```python
from build123d import *

# Parameters (mm, degrees)
SKETCH1_W           = 23
SKETCH1_H           = 23
BOSS_EXTRUDE1_DEPTH = 4
SKETCH2_W           = 11
SKETCH2_H           = 11
CUT_EXTRUDE1_DEPTH  = 4
SKETCH3_W           = 9
SKETCH3_H           = 4
BOSS_EXTRUDE2_DEPTH = 30


with BuildPart() as part:
    # Sketch1 → Boss-Extrude1 (new body)
    with BuildSketch(Plane(origin=(0, 0, 0), x_dir=(1, 0, 0), z_dir=(0, 1, 0))):
        with Locations((-0.318811881, 0.227722772)):
            Rectangle(SKETCH1_W, SKETCH1_H)
    extrude(amount=BOSS_EXTRUDE1_DEPTH)

    # Sketch2 → Cut-Extrude1 (cut)
    with BuildSketch(Plane(origin=(0, 4, 0), x_dir=(1, 0, 0), z_dir=(0, 1, 0))):
        with Locations((-0.318811881, 0.227722772)):
            Rectangle(SKETCH2_W, SKETCH2_H)
    extrude(amount=-CUT_EXTRUDE1_DEPTH, mode=Mode.SUBTRACT)

    # Sketch3 → Boss-Extrude2 (add)
    with BuildSketch(Plane(origin=(11.181188119, 0, 0), x_dir=(0, 0, -1), z_dir=(1, 0, 0))):
        with Locations((0.227722772, 2)):
            Rectangle(SKETCH3_W, SKETCH3_H)
    extrude(amount=BOSS_EXTRUDE2_DEPTH)


solid = part.part
```
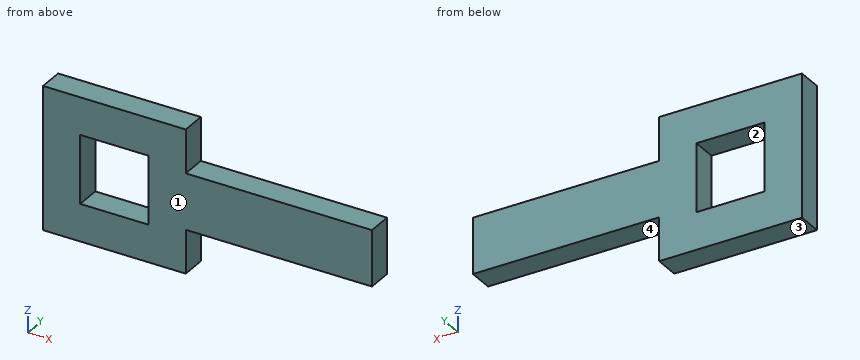
Work out the finished part from the listing and answer in its coordinate system (mm). Face numbers are marked on the shaded views. A direction names the side the tool comes from. Coordinates: 2 decimals unless noted, no trailing zeros. Write each loop counter-clockwise with the first axis right and the second up, starting at its lowest first coordinate (ties: lowest second). Pieces come first, ordered by that corner, then holes.
Q1. Determine the mould class of the marked faces 1 and 2 for opening direction X: released by +X, released by -X, zero draft, split by the parting line, or undercut.
Q2. A cutting plane is placed at D-D, the plane x = 36. Give the vertices of the cut face in (y, z).
Q3. A cutting plane is placed at C-C, the plane x = 1.5. Give the vertices of the cut face in (y, z).
Q4. This flat-tipped pin is pushed along its axis until it touches: pin 1 Ø1.2 at (x, y) = (30.5, 1) entering from -Z. Where does it stop, or does it pass through?
Q5. Which of the six approach directions +Z, -Z, +X, -X, +Y, -Y give full straight-line access (tool end or side, diameter ignored) to the marked faces 3 and 4?
Q6. A cutting plane is placed at A-A, the plane z = 2. Give the vertices of the cut face in (x, y).
Q7. A cutting plane is placed at B-B, the plane y = 0.7. Give the vertices of the cut face in (x, z).
Q8. Find the intervals of material crossed by line 1 (X direction, y = 1.95, z = -1.25); line 2 (Z direction, x = -2, y = 2.4); line 3 (X direction, y = 0.25, z = -5.25), in increasing order.
Findings below:
1. face 1: zero draft
1. face 2: undercut
2. outline: (0, -4.73) - (4, -4.73) - (4, 4.27) - (0, 4.27) - close
3. outline: (0, -11.73) - (4, -11.73) - (4, -5.73) - (0, -5.73) - close; (0, 5.27) - (4, 5.27) - (4, 11.27) - (0, 11.27) - close
4. pin 1: stops at z = -4.73
5. face 3: -Z, +X, -X, +Y, -Y
5. face 4: -Z, +X, +Y, -Y
6. outline: (-11.82, 0) - (-5.82, 0) - (-5.82, 4) - (-11.82, 4) - close; (5.18, 0) - (41.18, 0) - (41.18, 4) - (5.18, 4) - close
7. outline: (-11.82, -11.73) - (11.18, -11.73) - (11.18, -4.73) - (41.18, -4.73) - (41.18, 4.27) - (11.18, 4.27) - (11.18, 11.27) - (-11.82, 11.27) - close; hole (-5.82, -5.73) - (5.18, -5.73) - (5.18, 5.27) - (-5.82, 5.27) - close
8. line 1: x = -11.82 to -5.82, 5.18 to 41.18
8. line 2: z = -11.73 to -5.73, 5.27 to 11.27
8. line 3: x = -11.82 to -5.82, 5.18 to 11.18
